Work out the finished part from the listing and answer in its coordinate system (mm). Give positions to 0.01 mm unless a question says otherwise; leave off trailing zeros. Loops run counter-clockwise (first coordinate to the right, second up) from the corner with the lowest first, then second, coordinate; pieces in that order, holes last. Notation, with made-up numbers: (5, 82) - (12, 82) arc R26 ccw to (12, 121) - close; hole circle Ø10 at (-5, 47.25). An arc over 180 degrees is marked (long way). One line per question, with ' | ' between items.
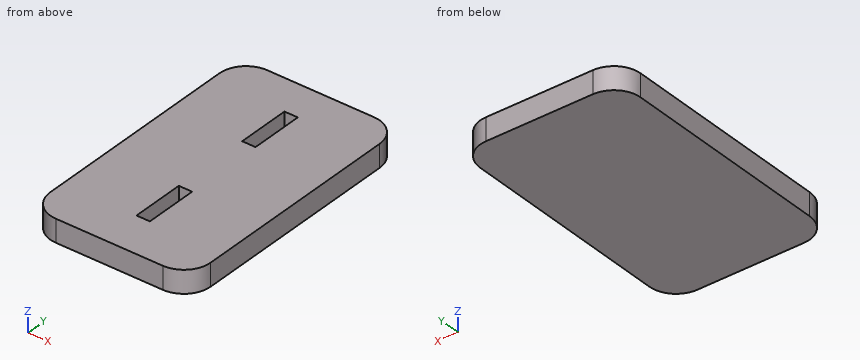
from build123d import *

# Parameters (mm, degrees)
CROQUIS2_W              = 60
CROQUIS2_H              = 100
SALIENTE_EXTRUIR1_DEPTH = 8.5
CROQUIS4_W              = 5
CROQUIS4_H              = 20
CORTAR_EXTRUIR1_DEPTH   = 7.48
REDONDEO1_R             = 10
REDONDEO2_R             = 10


with BuildPart() as part:
    # Croquis2 → Saliente-Extruir1 (new body)
    with BuildSketch(Plane.XY):
        Rectangle(CROQUIS2_W, CROQUIS2_H)
    extrude(amount=SALIENTE_EXTRUIR1_DEPTH)

    # Croquis4 → Cortar-Extruir1 (cut)
    with BuildSketch(Plane.XY.offset(8.5)):
        with Locations((0, 26.02)):
            Rectangle(CROQUIS4_W, CROQUIS4_H)
        with Locations((0, -23.98)):
            Rectangle(CROQUIS4_W, CROQUIS4_H)
    extrude(amount=-CORTAR_EXTRUIR1_DEPTH, mode=Mode.SUBTRACT)

    # Redondeo1
    redondeo1_edges = [part.edges().sort_by_distance(p)[0] for p in [
        (-30, 50, 4.25),
    ]]
    fillet(redondeo1_edges, radius=REDONDEO1_R)

    # Redondeo2
    redondeo2_edges = [part.edges().sort_by_distance(p)[0] for p in [
        (30, -50, 4.25),
        (-30, -50, 4.25),
        (30, 50, 4.25),
    ]]
    fillet(redondeo2_edges, radius=REDONDEO2_R)


solid = part.part
1. Find section C-C on y = -23.5. Write down the section's boundary in (x, z), then the cut area to 3 significant figures.
Evaluation:
outline: (-30, 0) - (30, 0) - (30, 8.5) - (2.5, 8.5) - (2.5, 1.02) - (-2.5, 1.02) - (-2.5, 8.5) - (-30, 8.5) - close | area: 473 mm2
2. Find section A-A on z = 5. Write down the section's boundary in (x, y).
Evaluation:
outline: (-30, -40) arc R10 ccw to (-20, -50) - (20, -50) arc R10 ccw to (30, -40) - (30, 40) arc R10 ccw to (20, 50) - (-20, 50) arc R10 ccw to (-30, 40) - close; hole (-2.5, -33.98) - (2.5, -33.98) - (2.5, -13.98) - (-2.5, -13.98) - close; hole (-2.5, 16.02) - (2.5, 16.02) - (2.5, 36.02) - (-2.5, 36.02) - close
3. Find section B-B on x = 1. Write down the section's boundary in (y, z), then the cut area to 3 significant figures.
Evaluation:
outline: (-50, 0) - (50, 0) - (50, 8.5) - (36.02, 8.5) - (36.02, 1.02) - (16.02, 1.02) - (16.02, 8.5) - (-13.98, 8.5) - (-13.98, 1.02) - (-33.98, 1.02) - (-33.98, 8.5) - (-50, 8.5) - close | area: 551 mm2
4. Find section D-D on x = 26. Write down the section's boundary in (y, z), then the cut area to 3 significant figures.
Evaluation:
outline: (-48, 0) - (48, 0) - (48, 8.5) - (-48, 8.5) - close | area: 816 mm2
5. Consider L1, parallel to Y at x = 0, z = 7.5; L2, parallel to X at y = -27, z = 8; L3, parallel to Y at x = 21, z = 4.5. Determine where each line is inside the solid, lowest interval first.
Evaluation:
L1: -50 to -33.98, -13.98 to 16.02, 36.02 to 50 | L2: -30 to -2.5, 2.5 to 30 | L3: -49.95 to 49.95
6. Flat-ended cylindrical pins translate along their axes: pin 1 (4 mm diameter, centred on x = 17, y = 0.5, fed in from -Z); pin 2 (1.5 mm diameter, centred on x = -1, y = -23.5, fed in from +Z). Find the tip coordinate at first contact, or state that the pin passes through.
Evaluation:
pin 1: z = 0 | pin 2: z = 1.02
